Autodesk Inventor part; units mm, degrees
ref_plane "YZ Plane" through (0, 0, 0) normal (1, 0, 0) x (0, 1, 0)
ref_plane "XZ Plane" through (0, 0, 0) normal (0, 1, 0) x (-1, 0, 0)
ref_plane "XY Plane" through (0, 0, 0) normal (0, 0, 1) x (1, 0, 0)
sketch "Sketch1" plane through (0, 0, 0) normal (0, 0, 1) x (1, 0, 0)
  line L0 (0, 0) -> (12.7, 0)
  line L1 (12.7, 0) -> (12.7, 38.1)
  line L2 (12.7, 38.1) -> (0, 38.1)
  line L3 (0, 38.1) -> (0, 0)
  line L4 (6.35, 0) -> (6.35, 6.35)
  line L5 (6.35, 6.35) -> (6.35, 31.75)
  circle A0 centre (6.35, 31.75) radius 2.54
  circle A1 centre (6.35, 6.35) radius 2.54
  dimension "d0" = 38.1
  dimension "d1" = 12.7
  dimension "d2" = 6.35
  dimension "d3" = 25.4
  dimension "d4" = 5.08
  dimension "d5" = 5.08
extrude "Extrusion1" add sketch "Sketch1" along normal blind 1.5875
fillet "Fillet1" radius 3.175 4 edges at (12.7, 0, 0.7937) (0, 0, 0.7937) (12.7, 38.1, 0.7937) (0, 38.1, 0.7937)
properties part number "polySpacer1"
Verification items for the finished model (mm, model axes). Give positions to 0.01 mm unless a question says otherwise; leave off trailing zeros. Order: outer loops, then holes, each group sorted by start corner. A loop starts at its lowest first (then second) coordinate and runs counter-clockwise, first axis right, second up. Notation, with made-up numbers: (40, 25) -> (45, 25) arc R37 ccw to (45, 62) -> close; hole circle Ø8 at (84.5, 87.25). An arc over 180 degrees is marked (long way). One line per item, written item: value.
(1) Sectioned sample at B-B on y = 6.35. Record the cut outline in (x, z).
Final values:
outline: (0, 0) -> (3.81, 0) -> (3.81, 1.59) -> (0, 1.59) -> close; (8.89, 0) -> (12.7, 0) -> (12.7, 1.59) -> (8.89, 1.59) -> close
(2) Sectioned sample at C-C on z = 0.75. Record the cut outline in (x, y) (3 decimals), then the cut area to 3 significant figures.
Final values:
outline: (0, 3.175) arc R3.175 ccw to (3.175, 0) -> (9.525, 0) arc R3.175 ccw to (12.7, 3.175) -> (12.7, 34.925) arc R3.175 ccw to (9.525, 38.1) -> (3.175, 38.1) arc R3.175 ccw to (0, 34.925) -> close; hole circle Ø5.08 at (6.35, 6.35); hole circle Ø5.08 at (6.35, 31.75)
area: 435 mm^2
(3) Draft check along X on faces 1 (the face through (6, 19, 0)), 2 (the face through (0.91, 0.95, 0.8)), 3 (the face through (6.02, 29.23, 0.78)). Enter one of: pulls with the +X half, pulls with the -X half, needs draft (parallel to the pull), parting line crosses it, or undercut.
Final values:
face 1: needs draft
face 2: pulls with the -X half
face 3: undercut
(4) Scan lines: line 1 along Y through (x, z) = (6.5, 0.4); line 2 along X through (y, z) = (31.75, 1.1); line 3 along Y through (x, z) = (7.25, 1). Record each from-to range of solid material in increasing order. Write a range as [from, to].
Final values:
line 1: [0, 3.81], [8.89, 29.21], [34.29, 38.1]
line 2: [0, 3.81], [8.89, 12.7]
line 3: [0, 3.97], [8.73, 29.37], [34.13, 38.1]
(5) Sectioned sample at A-A on x = 6.35. Record the cut outline in (y, z).
Final values:
outline: (0, 0) -> (3.81, 0) -> (3.81, 1.59) -> (0, 1.59) -> close; (8.89, 0) -> (29.21, 0) -> (29.21, 1.59) -> (8.89, 1.59) -> close; (34.29, 0) -> (38.1, 0) -> (38.1, 1.59) -> (34.29, 1.59) -> close
